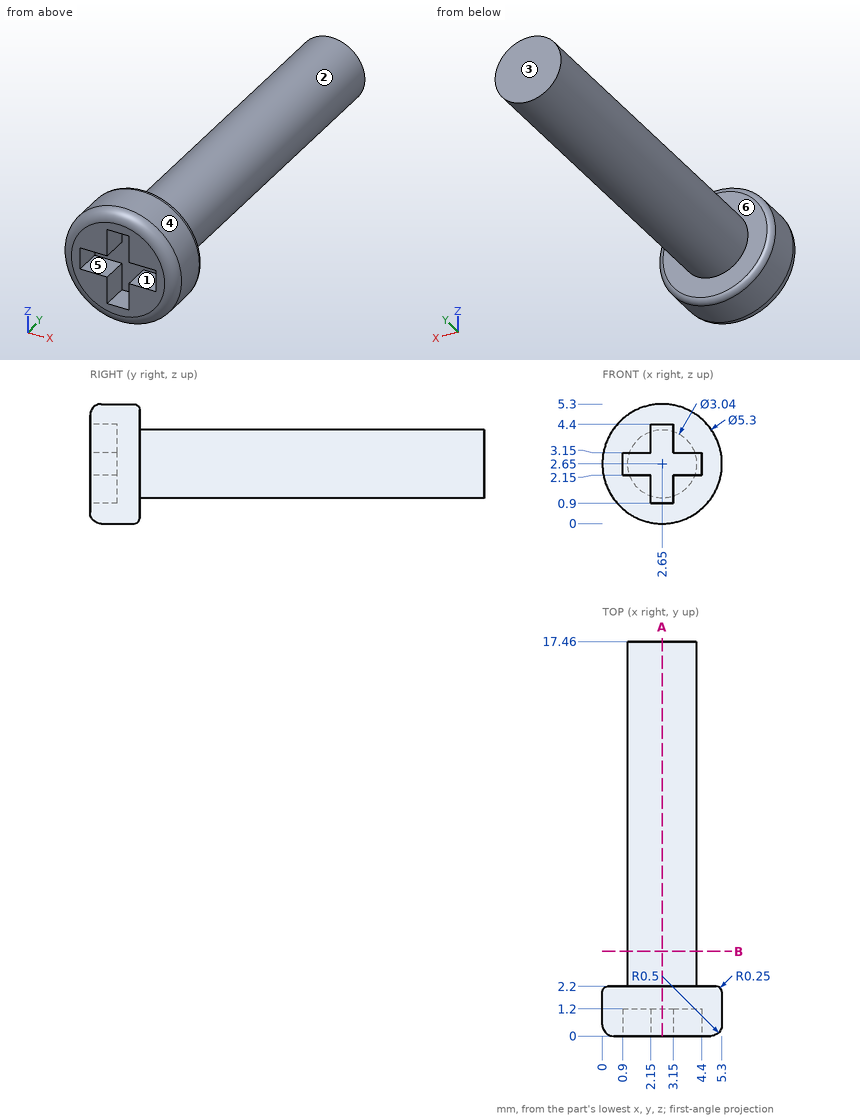
Check sheet for the drawn part. Datum: minimum x, y, z corner. Units: mm. A direction names the side the tool comes from. Round coordinates to 2 decimals unless told otherwise and drop trailing zeros. Order: outer loops, then holes, each group sorted by start corner. A loop starts at its lowest first (then second) coordinate and runs counter-clockwise, first axis right, second up. Notation, with made-up numbers: M -39,83 L -13,83 A9 cw -13,97 Z; hole C -32.5,-38 d2. An arc over 180 degrees is marked long. Write each question's results on one line, items separated by ' | '. Start each with the question number.
1. Set-up check for the marked faces 4, 5 and 6: record each of +Z, -Z, +X, -X, +Y, -Y from which the full face is reachable in a straight line by a thin tool's end or side.
2. Material ranges on L1, parallel to Y at x = 4.4, z = 3.9; L2, parallel to X at y = 11.75, z = 2.6; L3, parallel to Y at x = 2.6, z = 1.65, recorded low to high. Write a range as from..to.
3. Cross-section at B-B on y = 3.75. Record the boundary of the cut face in (x, z).
4. Draft check along Z on the marked faces 1, 2 and 3. Enter one of: pulls with the +Z half, pulls with the -Z half, needs draft (parallel to the pull), parting line crosses it, or undercut.
5. Cross-section at A-A on x = 2.65. Record the boundary of the cut face in (y, z).
6. Go/stop test with flat-tipped pins: P1, Ø1, axis at y = 0.5, z = 2, coming from the -X side; P2, Ø0.6, axis at y = 1, z = 3.5, coming from the +X side; P3, Ø1.5, axis at y = 7, z = 1.5, coming from the +X side. Record where each tip stops, or that it passes through.
Resolved:
1) face 4: +Y, -Y | face 5: -Y | face 6: +Y
2) L1: 0..2.2 | L2: 1.13..4.17 | L3: 1.2..17.46
3) outline: C 2.65,2.65 d3.04
4) face 1: undercut | face 2: parting line crosses it | face 3: needs draft
5) outline: M 0,0.5 A0.5 ccw 0.5,0 L 1.95,0 A0.25 ccw 2.2,0.25 L 2.2,1.13 L 17.46,1.13 L 17.46,4.17 L 2.2,4.17 L 2.2,5.05 A0.25 ccw 1.95,5.3 L 0.5,5.3 A0.5 ccw 0,4.8 L 0,4.4 L 1.2,4.4 L 1.2,0.9 L 0,0.9 Z
6) P1: x = 0 | P2: x = 5.24 | P3: x = 4.12
